Source: CAD feature listing. Evaluate the final solid. Frame: model axes, mm. Face numbers are marked on the shaded views. Coordinates: 2 decimals unless noted, no trailing zeros. Order: outer loops, then holes, each group sorted by start corner. A loop starts at its lowest first (then second) coordinate and runs counter-clockwise, first axis right, second up.
```python
from build123d import *

# Parameters (mm, degrees)
F0_W     = 1400
F0_H     = 700
F1_DEPTH = 25
F2_W     = 1400
F2_H     = 700
F2_W_2   = 1340
F2_H_2   = 640
F3_DEPTH = 37
F4_W     = 30
F4_H     = 30
F5_DEPTH = 690


with BuildPart() as f1:
    # F0 (on Top) → F1 (new body)
    with BuildSketch(Plane.XY):
        with Locations((700, -350)):
            Rectangle(F0_W, F0_H)
    extrude(amount=-F1_DEPTH)

    # F2 (on face) → F3 (join)
    with BuildSketch(Plane(origin=(0, 0, -25), x_dir=(1, 0, 0), z_dir=(0, 0, -1))):
        with Locations((700, 350)):
            Rectangle(F2_W, F2_H)
        with Locations((700, 350)):
            Rectangle(F2_W_2, F2_H_2, mode=Mode.SUBTRACT)
    extrude(amount=F3_DEPTH)

    # F4 (on face) → F5 (join)
    with BuildSketch(Plane(origin=(0, 0, -62), x_dir=(1, 0, 0), z_dir=(0, 0, -1))):
        with Locations((15, 685)):
            Rectangle(F4_W, F4_H)
        with Locations((15, 15)):
            Rectangle(F4_W, F4_H)
        with Locations((1385, 685)):
            Rectangle(F4_W, F4_H)
        with Locations((1385, 15)):
            Rectangle(F4_W, F4_H)
    extrude(amount=F5_DEPTH)


solid = f1.part
```
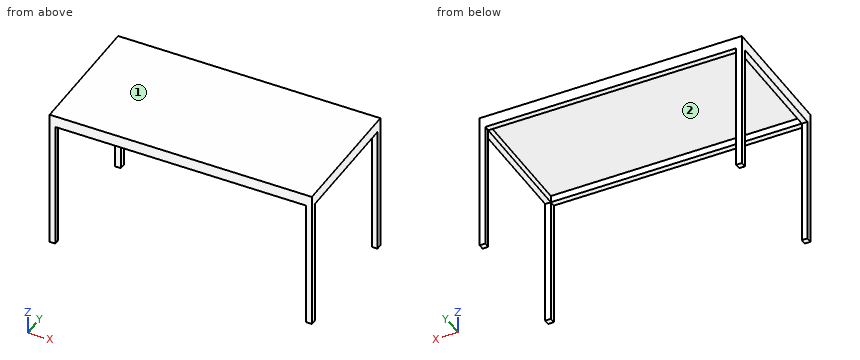
Q1. Section query A-A on z = -676.5. Output: boundary loops of the cut face in (x, y).
Solutions:
outline: (0, -700) - (30, -700) - (30, -670) - (0, -670) - close; (0, -30) - (30, -30) - (30, 0) - (0, 0) - close; (1370, -700) - (1400, -700) - (1400, -670) - (1370, -670) - close; (1370, -30) - (1400, -30) - (1400, 0) - (1370, 0) - close
Q2. Pull-direction query (Y, two-part tool) for the marked faces 1 and 2; classes: pulls with the +Y half, pulls with the -Y half, needs draft (parallel to the pull), parting line crosses it, or undercut.
Solutions:
face 1: needs draft
face 2: undercut
Q3. Section query B-B on x = 379. Output: boundary loops of the cut face in (y, z), plus the area to 3 significant figures.
Solutions:
outline: (-700, -62) - (-670, -62) - (-670, -25) - (-30, -25) - (-30, -62) - (0, -62) - (0, 0) - (-700, 0) - close
area: 19,700 mm2
Q4. Pin query (flat end, axial travel): P1, Ø9, axis at x = 822.5, y = -12, coming from the -Z side; P2, Ø8, axis at x = 754, y = -184.5, coming from the +Z side. Return the tip coordinate at first contact, or that it passes through.
Solutions:
P1: stops at z = -62
P2: stops at z = 0
Q5. Material intervals for line 1 along Y through (x, z) = (720, -30); line 2 along Z through (x, y) = (319, -421), sorted ascending.
Solutions:
line 1: y = -700 to -670, -30 to 0
line 2: z = -25 to 0
Q6. Section query C-C on y = -265. Output: boundary loops of the cut face in (x, z).
Solutions:
outline: (0, -62) - (30, -62) - (30, -25) - (1370, -25) - (1370, -62) - (1400, -62) - (1400, 0) - (0, 0) - close
